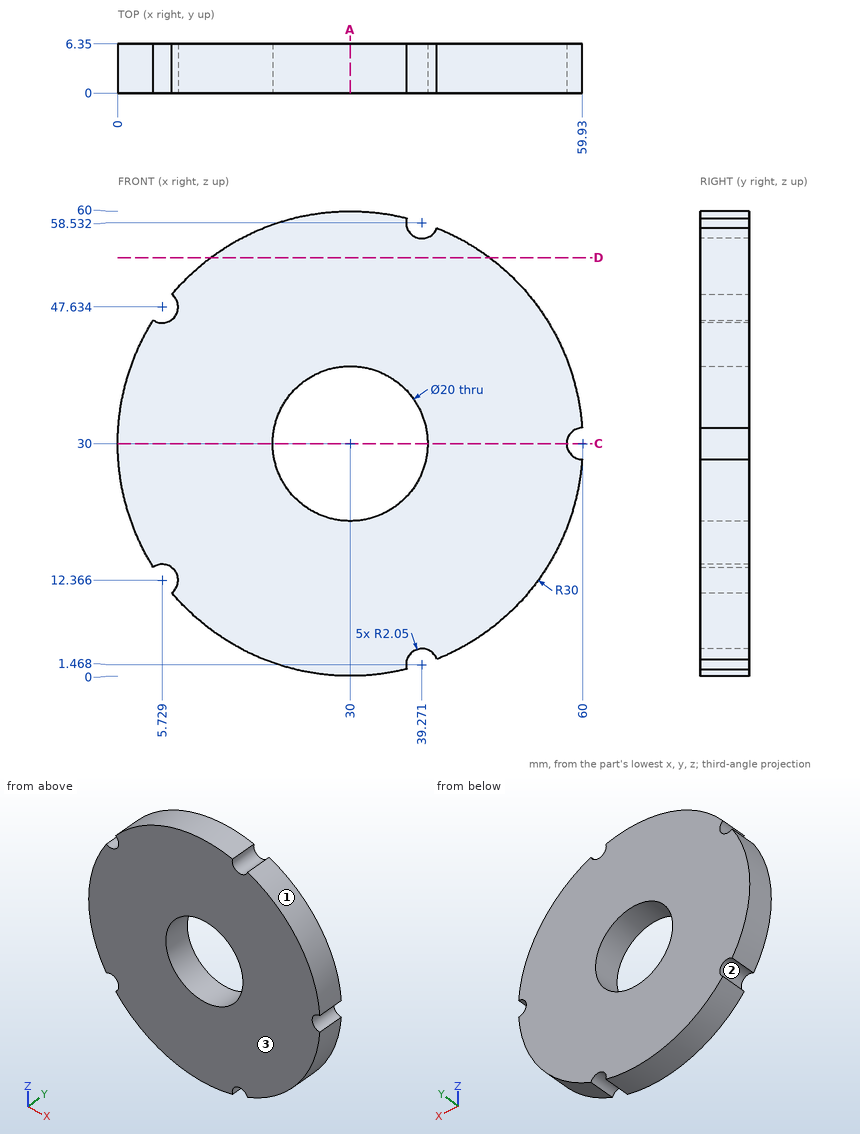
Geometry: see drawing. Coordinates: mm, zero at the bounding-box minimum. Give positions to 0.01 mm unless a question says otherwise; leave off trailing zeros. Order: outer loops, then holes, each group sorted by start corner. A loop starts at its lowest first (then second) coordinate and runs counter-clockwise, first axis right, second up.
1. Draft query along X for the marked faces 1, 2 and 3. Return one class per face: released by +X, released by -X, zero draft, split by the parting line, or undercut.
Computed:
face 1: released by +X
face 2: undercut
face 3: zero draft
2. Cut plane D-D (z = 54). Return loops of the section in (x, y), and give its area (3 significant figures).
Computed:
outline: (12, 0) - (48, 0) - (48, 6.35) - (12, 6.35) - close
area: 229 mm2
3. Line query: probe 1 along Z at (x, y) = (21, 1.5) (1 decimal); probe 2 along X at (y, z) = (1.25, 7); probe 3 along X at (y, z) = (1.75, 23). Output: solid intervals per line, ascending.
Computed:
probe 1: z = 1.4 to 25.6, 34.4 to 58.6
probe 2: x = 10.74 to 49.26
probe 3: x = 0.83 to 22.86, 37.14 to 59.17
4. Cut plane A-A (x = 30). Return loops of the section in (y, z).
Computed:
outline: (0, 0) - (6.35, 0) - (6.35, 20) - (0, 20) - close; (0, 40) - (6.35, 40) - (6.35, 60) - (0, 60) - close
5. Cut plane C-C (z = 30). Return loops of the section in (x, y), and give its area (3 significant figures).
Computed:
outline: (0, 0) - (20, 0) - (20, 6.35) - (0, 6.35) - close; (40, 0) - (57.95, 0) - (57.95, 6.35) - (40, 6.35) - close
area: 241 mm2
